```python
from build123d import *

# Parameters (mm, degrees)
SKETCH10_W          = 7
SKETCH10_H          = 6
SKETCH10_W_2        = 6
SKETCH10_H_2        = 7
BOSS_EXTRUDE4_DEPTH = 6
SKETCH11_R          = 1.5
CUT_EXTRUDE3_DEPTH  = 1.2
SKETCH14_R          = 1.5
CUT_EXTRUDE4_DEPTH  = 1.2
CUT_EXTRUDE5_START  = -1.2
SKETCH15_R          = 1.5
CUT_EXTRUDE5_DEPTH  = 1.2
CUT_EXTRUDE7_START  = -1.2
SKETCH16_R          = 1.5
CUT_EXTRUDE7_DEPTH  = 1.2
FILLET1_R           = 7
FILLET2_R           = 7
FILLET3_R           = 7
FILLET4_R           = 7
SKETCH17_R          = 1
CUT_EXTRUDE8_DEPTH  = 6


with BuildPart() as part:
    # Sketch10 → Boss-Extrude4 (new body)
    with BuildSketch(Plane.XY):
        with Locations((-272.368433777, 135.088329622)):
            Rectangle(SKETCH10_W, SKETCH10_H)
        with Locations((-265.868433777, 128.588329622)):
            Rectangle(SKETCH10_W_2, SKETCH10_H_2)
        with Locations((-259.368433777, 135.088329622)):
            Rectangle(SKETCH10_W, SKETCH10_H)
        with Locations((-265.868433777, 135.088329622)):
            Rectangle(SKETCH10_W_2, SKETCH10_H)
        with Locations((-265.868433777, 141.588329622)):
            Rectangle(SKETCH10_W_2, SKETCH10_H_2)
    extrude(amount=BOSS_EXTRUDE4_DEPTH)

    # Sketch11 → Cut-Extrude3 (cut)
    with BuildSketch(Plane(origin=(0, 145.088329622, 0), x_dir=(1, 0, 0), z_dir=(0, 1, 0))):
        with Locations(Location((-265.868433777, -3, 0), (0, 0, 270))):
            Circle(SKETCH11_R)
    extrude(amount=-CUT_EXTRUDE3_DEPTH, mode=Mode.SUBTRACT)

    # Sketch14 → Cut-Extrude4 (cut)
    with BuildSketch(Plane.ZY.offset(275.868433777)):
        with Locations((3, 135.088329622)):
            Circle(SKETCH14_R)
    extrude(amount=-CUT_EXTRUDE4_DEPTH, mode=Mode.SUBTRACT)

    # Sketch15 → Cut-Extrude5 (cut)
    with BuildSketch(Plane(origin=(0, 125.088329622, 0), x_dir=(-1, 0, 0), z_dir=(0, -1, 0)).offset(CUT_EXTRUDE5_START)):
        with Locations(Location((265.868433777, -3, 0), (0, 0, 270))):
            Circle(SKETCH15_R)
    extrude(amount=CUT_EXTRUDE5_DEPTH, mode=Mode.SUBTRACT)

    # Sketch16 → Cut-Extrude7 (cut)
    with BuildSketch(Plane(origin=(-255.868433777, 0, 0), x_dir=(0, 0, -1), z_dir=(1, 0, 0)).offset(CUT_EXTRUDE7_START)):
        with Locations(Location((-3, 135.088329622, 0), (0, 0, 180))):
            Circle(SKETCH16_R)
    extrude(amount=CUT_EXTRUDE7_DEPTH, mode=Mode.SUBTRACT)

    # Fillet1
    fillet1_edges = [part.edges().sort_by_distance(p)[0] for p in [
        (-262.868433777, 138.088329622, 3),
    ]]
    fillet(fillet1_edges, radius=FILLET1_R - 0.0001)  # a hair under: the kernel refuses the full size

    # Fillet2
    fillet2_edges = [part.edges().sort_by_distance(p)[0] for p in [
        (-268.868433777, 138.088329622, 3),
    ]]
    fillet(fillet2_edges, radius=FILLET2_R - 0.0001)  # a hair under: the kernel refuses the full size

    # Fillet3
    fillet3_edges = [part.edges().sort_by_distance(p)[0] for p in [
        (-268.868433777, 132.088329622, 3),
    ]]
    fillet(fillet3_edges, radius=FILLET3_R - 0.0001)  # a hair under: the kernel refuses the full size

    # Fillet4
    fillet4_edges = [part.edges().sort_by_distance(p)[0] for p in [
        (-262.868433777, 132.088329622, 3),
    ]]
    fillet(fillet4_edges, radius=FILLET4_R - 0.0001)  # a hair under: the kernel refuses the full size

    # Sketch17 → Cut-Extrude8 (cut)
    with BuildSketch(Plane(origin=(0, 0, 0), x_dir=(-1, 0, 0), z_dir=(0, 0, -1))):
        with Locations((265.868433777, 135.088329622)):
            Circle(SKETCH17_R)
    extrude(amount=-CUT_EXTRUDE8_DEPTH, mode=Mode.SUBTRACT)


solid = part.part
```
The model under review builds one solid part; all positions refer to its coordinate system, in mm. A direction names the side the tool comes from. Give positions to 0.01 mm unless a question says otherwise; leave off trailing zeros. Write each loop counter-clockwise with the first axis right and the second up, starting at its lowest first coordinate (ties: lowest second). Pieces come first, ordered by that corner, then holes.
(1) Consider section C-C, the plane y = 139.25. Give the boundary of the cut face in (x, z).
(2) To check wall thickness, follow L1, parallel to X at y = 135.25, z = 4.05; L2, parallel to Y at x = -256.75, z = 4.35; L3, parallel to Y at x = -274.95, z = 3. State the ranges of each line that lie inside material, in increasing order.
(3) For P1, Ø2.5, axis at y = 135.09, z = 3, coming from the -X side, flat-tipped, find the tip position at first contact; note if it passes through.
(4) Tool access review of faces 4 (the cylindrical face through (-267.2, 144.5, 3.69)), 5 (the flat face through (-257.068, 135, 3)), 6 (the cylindrical face through (-264.538, 125.697, 3.692)): name each direction out of +Z, -Z, +X, -X, +Y, -Y from which nothing blocks a thin tool from reaching the whole face with its end or side.
(5) The part is to be moulded in two halves that separate along Y. For faces 1 (the flat face through (-274.668, 135, 3)), 2 (the flat face through (-266, 137, 6)), 3 (the flat face through (-267.2, 145.088, 1.6)), say which applies: released by +Y, released by -Y, zero draft, split by the parting line, or undercut.
(6) Consider section B-B, the plane x = -271.5. Give the boundary of the cut face in (y, z).
Returned:
1. outline: (-272.01, 0) - (-259.73, 0) - (-259.73, 6) - (-272.01, 6) - close
2. L1: x = -274.67 to -266.86, -264.88 to -257.07
2. L2: y = 132.03 to 134.43, 135.74 to 138.14
2. L3: y = 132.03 to 133.59, 136.59 to 138.15
3. P1: stops at x = -274.67
4. face 4: +Y
4. face 5: +X
4. face 6: -Y
5. face 1: undercut
5. face 2: zero draft
5. face 3: released by +Y
6. outline: (130.56, 0) - (139.62, 0) - (139.62, 6) - (130.56, 6) - close
